Build history of the part. All positions in model axes, mm. Round coordinates to 2 decimals unless told otherwise and drop trailing zeros. Order: outer loops, then holes, each group sorted by start corner. A loop starts at its lowest first (then second) coordinate and runs counter-clockwise, first axis right, second up. Notation, with made-up numbers: (87, 18.5) -> (119, 18.5) arc R35 ccw to (119, 54.5) -> close; hole circle Ø11 at (65.5, 30.5). An arc over 180 degrees is marked (long way). Use a Markdown table: item, result. Add a question column.
Item 1: Slice it at A-A, the plane z = -1.1. Give the cut face in (x, y), plus the area to 3 significant figures.
Item 2: Slice it at B-B, the plane y = -44. Give the cut face in (x, z), plus the area to 3 significant figures.
Item 3: Two-plate mould, pull along Y, no slides. Class faces 1 (the face through (14, 1, 3)), 2 (the face through (-891.01, 5.26, 0.04)), 3 (the face through (983.883, 1.528, 0.042)): released by +Y, released by -Y, zero draft, split by the parting line, or undercut.
Item 4: Pin check, flat tips, straight feed: pin 1 (14.5 mm diameter, centred on x = 0, y = 0, fed in from -Z); pin 2 (3 mm diameter, centred on y = -52, z = 2.5, fed in from -X); pin 3 (1.5 mm diameter, centred on y = 46.5, z = -0.5, fed in from +X). Stop position of each tip, or through.
Item 5: Probe L1, parallel to Y at x = -907.7, z = -1.25; L2, parallel to Y at x = 0, z = 0.35; L3, parallel to X at y = -10, z = 1.75. List the from-to ranges inside material, lowest first.
from build123d import *

# Parameters (mm, degrees)
EXTRUDE_THIN1_DEPTH     = 3
BOSS_EXTRUDE1_DEPTH     = 3
SKETCH2_R               = 8
SKETCH2_R_2             = 17.5
CUT_EXTRUDE1_DEPTH      = 1
CUT_EXTRUDE1_DEPTH_BACK = 7


with BuildPart() as part:
    # Sketch1 → Extrude-Thin1 (new body, symmetric)
    with BuildSketch(Plane.XY):
        with BuildLine():
            Line((914.4, -69.5), (-914.4, -69.5))
            ThreePointArc((-914.4, -69.5), (-983.9, 0), (-914.4, 69.5))
            Line((-914.4, 69.5), (914.4, 69.5))
            ThreePointArc((914.4, 69.5), (983.9, 0), (914.4, -69.5))
        make_face()
        with BuildLine():
            Line((914.4, -63.5), (-914.4, -63.5))
            ThreePointArc((-914.4, -63.5), (-977.9, 0), (-914.4, 63.5))
            Line((-914.4, 63.5), (914.4, 63.5))
            ThreePointArc((914.4, 63.5), (977.9, 0), (914.4, -63.5))
        make_face(mode=Mode.SUBTRACT)
    extrude(amount=EXTRUDE_THIN1_DEPTH, both=True)

    # Sketch1<3> → Boss-Extrude1 (add, symmetric)
    with BuildSketch(Plane.XY):
        with BuildLine():
            Line((-914.4, 63.5), (914.4, 63.5))
            ThreePointArc((914.4, 63.5), (977.9, 0), (914.4, -63.5))
            Line((914.4, -63.5), (-914.4, -63.5))
            ThreePointArc((-914.4, -63.5), (-977.9, 0), (-914.4, 63.5))
        make_face()
    extrude(amount=BOSS_EXTRUDE1_DEPTH, both=True)

    # Sketch2 → Cut-Extrude1 (cut, two sides)
    with BuildSketch(Plane.XY.offset(3)) as cut_extrude1_sk:
        Circle(SKETCH2_R)
        with Locations((907.7, 0)):
            Circle(SKETCH2_R)
        with Locations((-907.7, 0)):
            Circle(SKETCH2_R_2)
        with Locations((453.85, 0)):
            Circle(SKETCH2_R)
        with Locations((-453.85, 0)):
            Circle(SKETCH2_R)
    extrude(amount=CUT_EXTRUDE1_DEPTH, mode=Mode.SUBTRACT)
    extrude(cut_extrude1_sk.sketch, amount=-CUT_EXTRUDE1_DEPTH_BACK, mode=Mode.SUBTRACT)


solid = part.part
Check sheet entries:
| question | item | result |
|---|---|---|
| 1 | outline | (-914.4, -69.5) -> (914.4, -69.5) arc R69.5 ccw to (914.4, 69.5) -> (-914.4, 69.5) arc R69.5 ccw to start; hole circle Ø35 at (-907.7, 0); hole circle Ø16 at (-453.85, 0); hole circle Ø16 at (0, 0); hole circle Ø16 at (453.85, 0); hole circle Ø16 at (907.7, 0) |
| 1 | area | 268,000 mm2 |
| 2 | outline | (-968.2, -3) -> (968.2, -3) -> (968.2, 3) -> (-968.2, 3) -> close |
| 2 | area | 11,600 mm2 |
| 3 | face 1 | zero draft |
| 3 | face 2 | undercut |
| 3 | face 3 | split by the parting line |
| 4 | pin 1 | through |
| 4 | pin 2 | x = -962.15 |
| 4 | pin 3 | x = 966.72 |
| 5 | L1 | -69.5 to -17.5, 17.5 to 69.5 |
| 5 | L2 | -69.5 to -8, 8 to 69.5 |
| 5 | L3 | -983.18 to -922.06, -893.34 to 983.18 |
